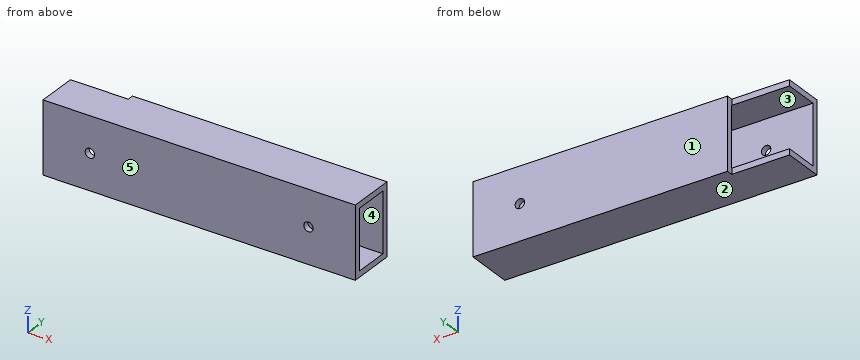
from build123d import *

# Parameters (mm, degrees)
SKETCH_1_W          = 100
SKETCH_1_H          = 19
SKETCH_1_R          = 1.5
EXTRUDE_2_DEPTH     = 2
SKETCH_2_W          = 100
SKETCH_2_H          = 2
EXTRUDE_3_DEPTH     = 15
SKETCH_3_W          = 100
SKETCH_3_H          = 19
SKETCH_3_R          = 1.5
EXTRUDE_5_DEPTH     = 2
CUT_EXTRUDE_1_DEPTH = 2
SKETCH_7_W          = 19
SKETCH_7_H          = 11
CUT_EXTRUDE_2_DEPTH = 100
CUT_EXTRUDE_3_DEPTH = 2


with BuildPart() as part:
    # 草图1 → 凸台-拉伸2 (new body)
    with BuildSketch(Plane(origin=(0, 0, 0), x_dir=(1, 0, 0), z_dir=(0, 1, 0))):
        Rectangle(SKETCH_1_W, SKETCH_1_H)
        with Locations(Location((-35, 0, 0), (0, 0, 270))):
            Circle(SKETCH_1_R, mode=Mode.SUBTRACT)
        with Locations(Location((35, 0, 0), (0, 0, 270))):
            Circle(SKETCH_1_R, mode=Mode.SUBTRACT)
    extrude(amount=EXTRUDE_2_DEPTH)

    # 草图2 → 凸台-拉伸3 (add)
    with BuildSketch(Plane(origin=(0, 2, 0), x_dir=(1, 0, 0), z_dir=(0, 1, 0))):
        with Locations((0, -10.5)):
            Rectangle(SKETCH_2_W, SKETCH_2_H)
        with Locations((0, 10.5)):
            Rectangle(SKETCH_2_W, SKETCH_2_H)
    extrude(amount=-EXTRUDE_3_DEPTH)

    # 草图3 → 凸台-拉伸5 (add)
    with BuildSketch(Plane(origin=(0, -13, 0), x_dir=(-1, 0, 0), z_dir=(0, -1, 0))):
        Rectangle(SKETCH_3_W, SKETCH_3_H)
        with Locations(Location((35, 0, 0), (0, 0, 270))):
            Circle(SKETCH_3_R, mode=Mode.SUBTRACT)
        with Locations(Location((-35, 0, 0), (0, 0, 270))):
            Circle(SKETCH_3_R, mode=Mode.SUBTRACT)
    extrude(amount=-EXTRUDE_5_DEPTH)

    # 草图5 → 切除-拉伸1 (cut)
    with BuildSketch(Plane(origin=(0, 2, 0), x_dir=(1, 0, 0), z_dir=(0, 1, 0))):
        Polygon((-38.5, -11.5), (-38.5, 0), (-38.5, 11.5), (-50, 11.5), (-50, -11.5), align=None)
    extrude(amount=-CUT_EXTRUDE_1_DEPTH, mode=Mode.SUBTRACT)

    # 草图7 → 切除-拉伸2 (cut)
    with BuildSketch(Plane(origin=(50, 0, 0), x_dir=(0, 0, -1), z_dir=(1, 0, 0))):
        Polygon((9.5, 0), (9.5, -11), (9.6, -11), (9.6, 0.1), (-9.5, 0.1), (-9.5, 0), align=None)
        with Locations((0, -5.5)):
            Rectangle(SKETCH_7_W, SKETCH_7_H)
        Polygon((-9.6, 0.1), (-9.6, -11.1), (9.6, -11.1), (9.6, -11), (9.5, -11), (-9.5, -11), (-9.5, 0), (-9.5, 0.1), align=None)
    extrude(amount=-CUT_EXTRUDE_2_DEPTH, mode=Mode.SUBTRACT)

    # 草图8 → 切除-拉伸3 (cut)
    with BuildSketch(Plane(origin=(0, 2, 0), x_dir=(1, 0, 0), z_dir=(0, 1, 0))):
        Polygon((-31.5, -11.5), (-31.5, 0), (-31.5, 11.5), (-38.5, 11.5), (-38.5, -11.5), align=None)
    extrude(amount=-CUT_EXTRUDE_3_DEPTH, mode=Mode.SUBTRACT)


solid = part.part
Read the model definition and answer for the solid it produces. Units are mm, in the model's axes. Face numbers are marked on the shaded views. A direction names the side the tool comes from. Coordinates: 2 decimals unless noted, no trailing zeros. Order: outer loops, then holes, each group sorted by start corner. A loop starts at its lowest first (then second) coordinate and runs counter-clockwise, first axis right, second up. Notation, with made-up numbers: M -23,52.5 L -11,52.5 A22 ccw -11,75.5 Z; hole C -23,61.25 d11. An arc over 180 degrees is marked long. Put each result on its own line as item: value. Start each with the question number.
Item 1: Consider probe 1 along X at (y, z) = (-11.6, 0); probe 2 along Z at (x, y) = (24.5, -1.25); probe 3 along Y at (x, z) = (23.5, -2). Determine where each line is inside the solid, lowest interval first. Write a range as [from, to].
Item 2: Section D-D, the plane z = 0 is taken. Determine the outline of the cut face in (x, y), plus the area to 3 significant figures.
Item 3: Section A-A, the plane z = 6.75 is taken. Determine the outline of the cut face in (x, y).
Item 4: Section B-B, the plane y = -8.5 is taken. Determine the outline of the cut face in (x, z).
Item 5: Section C-C, the plane x = -35 is taken. Determine the outline of the cut face in (y, z), plus the area to 3 significant figures.
Item 6: The mould has two halves that part along Y. Classify the marked faces 1, 2 and 3: +Y half, -Y half, draft (parallel to the pull), parting line (faces both ways), or undercut.
Item 7: For the marked faces 4 and 5, determine the directions among +Z, -Z, +X, -X, +Y, -Y from which every point of the face is accessible in a straight line to the end or side of a thin tool.
Item 8: Given pin 1 Ø1 at (y, z) = (-11, 0.5) entering from +X; pin 2 Ø1 at (y, z) = (1, 4.5) entering from -X; pin 3 Ø1 at (x, z) = (-42, -10.5) entering from +Y, each flat-ended and moving along its own axis, determine where each tip first touches the part or whether it passes through.
Computed:
1. probe 1: x = [-50, -36.5], [-33.5, 33.5], [36.5, 50]
1. probe 2: z = [-11.5, -9.6], [9.6, 11.5]
1. probe 3: y = [-13, -11.1], [0.1, 2]
2. outline: M -50,-13 L -36.5,-13 L -36.5,-11.1 L -50,-11.1 Z; M -33.5,-13 L 33.5,-13 L 33.5,-11.1 L -33.5,-11.1 Z; M -31.5,0.1 L 33.5,0.1 L 33.5,2 L -31.5,2 Z; M 36.5,-13 L 50,-13 L 50,-11.1 L 36.5,-11.1 Z; M 36.5,0.1 L 50,0.1 L 50,2 L 36.5,2 Z
2. area: 328 mm2
3. outline: M -50,-13 L 50,-13 L 50,-11.1 L -50,-11.1 Z; M -31.5,0.1 L 50,0.1 L 50,2 L -31.5,2 Z
4. outline: M -50,-11.5 L 50,-11.5 L 50,-9.6 L -50,-9.6 Z; M -50,9.6 L 50,9.6 L 50,11.5 L -50,11.5 Z
5. outline: M -13,-11.5 L 0,-11.5 L 0,-9.6 L -11.1,-9.6 L -11.1,-1.5 L -13,-1.5 Z; M -13,1.5 L -11.1,1.5 L -11.1,9.6 L 0,9.6 L 0,11.5 L -13,11.5 Z
5. area: 80.2 mm2
6. face 1: +Y half
6. face 2: draft
6. face 3: undercut
7. face 4: +X, -X
7. face 5: +Z, -Z, +X, -X, -Y
8. pin 1: stops at x = 50
8. pin 2: stops at x = -31.5
8. pin 3: stops at y = 0
